Design review of the part shown in the three views and the two pictorial views. Dimensions are in mm from the part's minimum x, y and z. A direction names the side the tool comes from. Round coordinates to 2 decimals unless told otherwise and drop trailing zeros. Order: outer loops, then holes, each group sorted by start corner. A loop starts at its lowest first (then second) coordinate and runs counter-clockwise, first axis right, second up. Notation, with made-up numbers: M -14,43 L -5,43 A27 cw -5,70 Z; hole C 89,15.5 d3. An arc over 180 degrees is marked long. Write each question's results on one line, items separated by ' | '. Start each with the question number.
Item 1: The part is to be moulded in two halves that separate along X. For the marked faces 1, 2 and 3, say which applies: +X half, -X half, draft (parallel to the pull), parting line (faces both ways), or undercut.
Item 2: Take a section at A-A, the plane z = 4. Write out the cut boundary in (x, y), plus the area to 3 significant figures.
Item 3: Take a section at D-D, the plane x = 18. Write out the cut boundary in (y, z).
Item 4: Clearance check with flat-ended pins moving along their axes: pin 1 (8 mm diameter, centred on x = 16.5, z = 10.5, fed in from +Y); pin 2 (3 mm diameter, centred on x = 11.5, y = 2.5, fed in from +Z); pin 3 (3.5 mm diameter, centred on x = 14.5, y = 8, fed in from -Z); pin 4 (5 mm diameter, centred on x = 12.5, z = 16.5, fed in from +Y). State where each tip first meets the part, or that it passes through.
Item 5: Take a section at B-B, the plane x = 8. Write out the cut boundary in (y, z).
Item 6: Take a section at C-C, the plane y = 2.75. Write out the cut boundary in (x, z), plus the area to 3 significant figures.
Item 7: Machinability: for the marked faces 4, 5, 6 and 7, which of the approach directions +Z, -Z, +X, -X, +Y, -Y give a long, thin tool a straight path to every point of the face, cutting with its end or side? Answer none if there is none.
Item 8: Wall thickness on line 1 (X direction, y = 4.5, z = 26); line 2 (Y direction, x = 10.5, z = 28); line 3 (Z direction, x = 3.5, y = 13.75): over which ranges is each line inside the solid? List them lowest first. Write a range as [from, to].
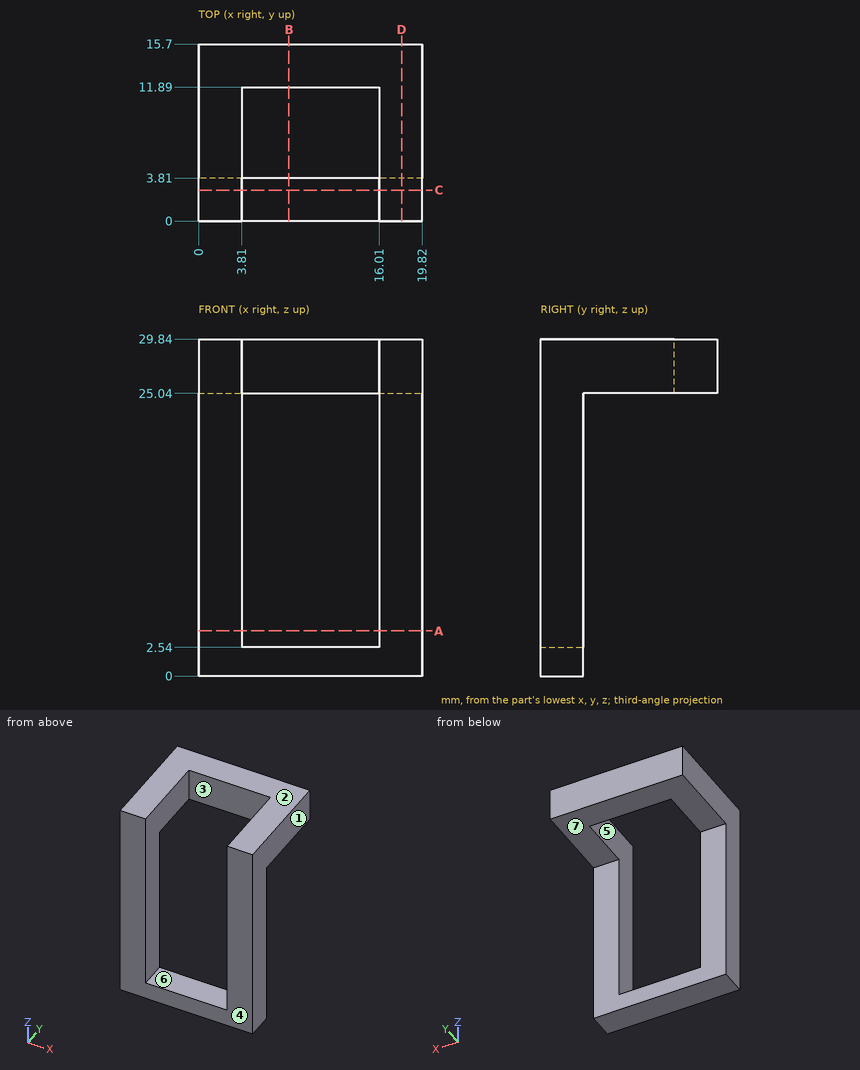
Results list:
1) face 1: +X half | face 2: draft | face 3: undercut
2) outline: M 0,0 L 3.81,0 L 3.81,3.81 L 0,3.81 Z; M 16.01,0 L 19.82,0 L 19.82,3.81 L 16.01,3.81 Z | area: 29.0 mm²
3) outline: M 0,0 L 3.81,0 L 3.81,25.04 L 15.7,25.04 L 15.7,29.84 L 0,29.84 Z
4) pin 1: y = 3.81 | pin 2: z = 2.54 | pin 3: z = 25.04 | pin 4: through
5) outline: M 0,0 L 3.81,0 L 3.81,2.54 L 0,2.54 Z; M 11.89,25.04 L 15.7,25.04 L 15.7,29.84 L 11.89,29.84 Z
6) outline: M 0,0 L 19.82,0 L 19.82,29.84 L 16.01,29.84 L 16.01,2.54 L 3.81,2.54 L 3.81,29.84 L 0,29.84 Z | area: 258 mm²
7) face 4: +Z, -Z, +X, -X, -Y | face 5: +Z, -Y | face 6: +Z, +Y, -Y | face 7: -Z, +X, -X, +Y
8) line 1: [0, 3.81], [16.01, 19.82] | line 2: [11.89, 15.7] | line 3: [25.04, 29.84]
